Can you work these out from the model? Positions are in its coordinate system, mm. A direction names the side the tool comes from. Give positions to 0.01 mm unless a question says otherwise; leave off trailing zeros. Loops run counter-clockwise (first coordinate to the right, second up) from the corner with the lowest first, then second, coordinate; pieces in that order, holes last. Notation, with made-up numbers: (-1, -12) - (16, -12) arc R3 ccw to (16, -8) - close; hole circle Ø9 at (7.25, -11.5). An arc over 180 degrees is marked (long way). Use a Markdown table: item, result. Add a question column.
```python
from build123d import *

# Parameters (mm, degrees)
SKETCH_1_R          = 3
SKETCH_1_W          = 12.5
SKETCH_1_H          = 23.5
EXTRUDE_1_DEPTH     = 5
SKETCH_2_W          = 12.5
SKETCH_2_H          = 4.75
SKETCH_2_R          = 1.25
EXTRUDE_2_DEPTH     = 17
SKETCH_4_R          = 25
EXTRUDE_7_DEPTH     = 4
SKETCH_5_W          = 8.371461974
SKETCH_5_H          = 5.334847295
CUT_EXTRUDE_1_DEPTH = 42
FILLET_1_R          = 2
SKETCH_6_R          = 4.21665728
CUT_EXTRUDE_2_DEPTH = 10


with BuildPart() as part:
    # 草图1 → 凸台-拉伸1 (new body)
    with BuildSketch(Plane(origin=(0, 0, 0), x_dir=(1, 0, 0), z_dir=(0, 1, 0))):
        with BuildLine():
            Line((27, 30), (-27, 30))
            ThreePointArc((-27, 30), (-29.121320344, 29.121320344), (-30, 27))
            Line((-30, 27), (-30, -27))
            ThreePointArc((-30, -27), (-29.121320344, -29.121320344), (-27, -30))
            Line((-27, -30), (27, -30))
            ThreePointArc((27, -30), (29.121320344, -29.121320344), (30, -27))
            Line((30, -27), (30, 27))
            ThreePointArc((30, 27), (29.121320344, 29.121320344), (27, 30))
        make_face()
        with Locations((-23, 23)):
            Circle(SKETCH_1_R, mode=Mode.SUBTRACT)
        with Locations((23, 23)):
            Circle(SKETCH_1_R, mode=Mode.SUBTRACT)
        with Locations((23, -23)):
            Circle(SKETCH_1_R, mode=Mode.SUBTRACT)
        with Locations((-23, -23)):
            Circle(SKETCH_1_R, mode=Mode.SUBTRACT)
        with Locations((0, 5.5)):
            Rectangle(SKETCH_1_W, SKETCH_1_H, mode=Mode.SUBTRACT)
    extrude(amount=EXTRUDE_1_DEPTH)

    # 草图2 → 凸台-拉伸2 (add)
    with BuildSketch(Plane(origin=(0, 5, 0), x_dir=(1, 0, 0), z_dir=(0, 1, 0))):
        with Locations((0, 19.625)):
            Rectangle(SKETCH_2_W, SKETCH_2_H)
        with Locations((0, 19)):
            Circle(SKETCH_2_R, mode=Mode.SUBTRACT)
        with Locations((0, -8.625)):
            Rectangle(SKETCH_2_W, SKETCH_2_H)
        with Locations((0, -8)):
            Circle(SKETCH_2_R, mode=Mode.SUBTRACT)
    extrude(amount=EXTRUDE_2_DEPTH)

    # 草图4 → 凸台-拉伸7 (add)
    with BuildSketch(Plane(origin=(0, 5, 0), x_dir=(1, 0, 0), z_dir=(0, 1, 0))):
        Circle(SKETCH_4_R)
        with BuildLine():
            Line((-6.285373074, 22.124513222), (-6.25, 22))
            Line((-6.25, 22), (6.25, 22))
            Line((6.25, 22), (6.285373074, 22.124513222))
            ThreePointArc((6.285373074, 22.124513222), (0, -23), (-6.285373074, 22.124513222))
        make_face(mode=Mode.SUBTRACT)
    extrude(amount=EXTRUDE_7_DEPTH)

    # 草图5 → 切除-拉伸1 (cut)
    with BuildSketch(Plane.XY.offset(11)):
        with Locations((0, 7.667423648)):
            Rectangle(SKETCH_5_W, SKETCH_5_H)
    extrude(amount=-CUT_EXTRUDE_1_DEPTH, mode=Mode.SUBTRACT)

    # 圆角1
    fillet_1_edges = [part.edges().sort_by_distance(p)[0] for p in [
        (-4.185730987, 7, -24.647102388),
        (4.185730987, 7, -24.647102388),
    ]]
    fillet(fillet_1_edges, radius=FILLET_1_R)

    # 草图6 → 切除-拉伸2 (cut)
    with BuildSketch(Plane(origin=(0, 5, 0), x_dir=(1, 0, 0), z_dir=(0, 1, 0))):
        with Locations((-14.961939604, 0)):
            Circle(SKETCH_6_R)
    extrude(amount=-CUT_EXTRUDE_2_DEPTH, mode=Mode.SUBTRACT)


solid = part.part
```
1. On a 3-axis mill with a long thin cutter (end or side, diameter ignored), from which of +Z, -Z, +X, -X, +Y, -Y can I reach the whole of each face in a straight line? I mean faces 4 (the face through (0, 11, 6.25)), 5 (the face through (0.92, 6.97, 22.98)), 6 (the face through (4.186, 8, 9)), 7 (the face through (0, 10.335, -21)). Say none if no direction works.
2. Suppose I cut it at B-B (x = 0). List the corners of the cut face in (y, z) for me.
3. Will these pins go through, and if not, where does the flat tip stop? P1, Ø2, axis at y = 6.5, z = 16.5, coming from the -X side; P2, Ø5, axis at x = 23, z = 23, coming from the -Y side; P3, Ø2.5, axis at y = 17, z = 9.5, coming from the -X side; P4, Ø6, axis at y = 11, z = -7.5, coming from the -X side.
4. Suppose I cut it at D-D (z = -16). List the corners of the cut face in (x, y) for me.
5. Please list where these lines run through material, in increasing order: line 1 along X through (y, z) = (3.75, 0); line 2 along Z through (x, y) = (0, 19); line 3 along X through (y, z) = (2.8, -23). Write a range as [from, to].
6. Suppose I cut it at A-A (y = 18.25). List the corners of the cut face in (x, z) for me, and give its area (3 significant figures).
7. If we mould it in two halves opening along Z, with no side actions, what happens to faces 1 (the face through (4.997, 6.972, -23.761)), 2 (the face through (6.25, 2, -5)), 3 (the face through (7.3, 9, 22.2))? For each: released by +Z, released by -Z, zero draft, split by the parting line, or undercut.
8. Suppose I cut it at C-C (y = 1.5). List the corners of the cut face in (x, z) for me.
Results below:
| question | item | result |
|---|---|---|
| 1 | face 4 | +Y, -Y |
| 1 | face 5 | +Y |
| 1 | face 6 | -Z |
| 1 | face 7 | +Z, -Z |
| 2 | outline | (0, -30) - (5, -30) - (5, -17.25) - (0, -17.25) - close; (0, 6.25) - (5, 6.25) - (5, 23) - (9, 23) - (9, 25) - (5, 25) - (5, 30) - (0, 30) - close; (10.33, -22) - (22, -22) - (22, -20.25) - (10.33, -20.25) - close; (10.33, -17.75) - (22, -17.75) - (22, -17.25) - (10.33, -17.25) - close; (10.33, 6.25) - (22, 6.25) - (22, 6.75) - (10.33, 6.75) - close; (10.33, 9.25) - (22, 9.25) - (22, 11) - (10.33, 11) - close |
| 3 | P1 | x = -19.62 |
| 3 | P2 | through |
| 3 | P3 | x = -6.25 |
| 3 | P4 | x = -24.44 |
| 4 | outline | (-30, 0) - (-6.25, 0) - (-6.25, 5) - (-16.52, 5) - (-16.52, 9) - (-19.21, 9) - (-19.21, 5) - (-30, 5) - close; (6.25, 0) - (30, 0) - (30, 5) - (19.21, 5) - (19.21, 9) - (16.52, 9) - (16.52, 5) - (6.25, 5) - close |
| 5 | line 1 | [-30, -19.18], [-10.75, -6.25], [6.25, 30] |
| 5 | line 2 | [-22, -20.25], [-17.75, -17.25], [6.25, 6.75], [9.25, 11] |
| 5 | line 3 | [-30, -26], [-20, 20], [26, 30] |
| 6 | outline | (-6.25, -22) - (6.25, -22) - (6.25, -17.25) - (-6.25, -17.25) - close; (-6.25, 6.25) - (6.25, 6.25) - (6.25, 11) - (-6.25, 11) - close; hole circle Ø2.5 at (0, -19); hole circle Ø2.5 at (0, 8) |
| 6 | area | 109 mm² |
| 7 | face 1 | released by -Z |
| 7 | face 2 | undercut |
| 7 | face 3 | zero draft |
| 8 | outline | (-30, -27) arc R3 ccw to (-27, -30) - (27, -30) arc R3 ccw to (30, -27) - (30, 27) arc R3 ccw to (27, 30) - (-27, 30) arc R3 ccw to (-30, 27) - close; hole circle Ø6 at (-23, -23); hole circle Ø6 at (-23, 23); hole circle Ø8.43 at (-14.96, 0); hole (-6.25, -17.25) - (6.25, -17.25) - (6.25, 6.25) - (-6.25, 6.25) - close; hole circle Ø6 at (23, -23); hole circle Ø6 at (23, 23) |
